Verification items for the finished model (mm, model axes). A direction names the side the tool comes from. Round coordinates to 2 decimals unless told otherwise and drop trailing zeros. Write each loop counter-clockwise with the first axis right and the second up, starting at its lowest first coordinate (ties: lowest second). Pieces come first, ordered by that corner, then holes. Notation, with made-up numbers: M 75,68 L 90,68 A25 ccw 90,85 Z; hole C -2,-28.5 d10. An arc over 180 degrees is marked long. One line per question, with ' | ' between items. Start each with the question number.
Q1. Cross-section at C-C (x = 86). Record the boundary of the cut face in (y, z).
Q2. Thickness scan on line 1 along X through (y, z) = (40, 11.3); line 2 along Y through (x, z) = (55, 12.5); line 3 along X through (y, z) = (88, 11.15). Record the ranges inside material, lowest first. Write a range as from..to.
Q3. Tool access check on faces 1 (the face through (172, 40, 5)), 2 (the face through (85, 76.5, 6)), 3 (the face through (101, 82, 10)). Record the directions out of +Z, -Z, +X, -X, +Y, -Y that give a thin tool (end or side, any length) a straight path to the whole face; none if there is none.
Q4. Cross-section at B-B (y = 40). Record the boundary of the cut face in (x, z).
Q5. Cross-section at A-A (x = 46). Record the boundary of the cut face in (y, z), then the cut area to 4 significant figures.
Q6. Gauge pin test, flat ends, axial feed: pin 1 (5 mm diameter, centred on y = 36.5, z = 5, fed in from -X); pin 2 (11 mm diameter, centred on x = 86, y = -8, fed in from -Z); pin 3 (1.5 mm diameter, centred on y = 55, z = 9, fed in from +X). Record the tip position at first contact, or that the pin passes through.
Q7. Cross-section at D-D (z = 5.75). Record the boundary of the cut face in (x, y), then the cut area to 4 significant figures.
Q8. Release check for a two-part mould opening along X. For faces 4 (the face through (85, 0, 5)), 5 (the face through (-13.15, 92.99, 11.52)), 6 (the face through (180, 40, 12)) record: released by +X, released by -X, zero draft, split by the parting line, or undercut.
from build123d import *

# Parameters (mm, degrees)
ESQUISSE1_W                  = 172
ESQUISSE1_H                  = 80
ESQUISSE1_W_2                = 165
ESQUISSE1_H_2                = 73
BOSS_EXTRU_1_DEPTH           = 10
ESQUISSE2_W                  = 204
ESQUISSE2_H                  = 112
ESQUISSE2_W_2                = 165
ESQUISSE2_H_2                = 73
BOSS_EXTRU_2_DEPTH           = 3
CONG_1_R                     = 10
CONG_2_R                     = 5
ENL_V_MAT_EXTRU_1_DEPTH      = 212.329127193
ENL_V_MAT_EXTRU_1_DEPTH_BACK = 2
ESQUISSE3_R                  = 3.5
ENL_V_MAT_EXTRU_2_DEPTH      = 212.492316645
ENL_V_MAT_EXTRU_2_DEPTH_BACK = 212.492316645
ESQUISSE4_R                  = 2
CHANFREIN1_SIZE              = 1.5


with BuildPart() as part:
    # Esquisse1 → Boss.-Extru.1 (new body)
    with BuildSketch(Plane.XY):
        with Locations((86, 40)):
            Rectangle(ESQUISSE1_W, ESQUISSE1_H)
        with Locations((86, 40)):
            Rectangle(ESQUISSE1_W_2, ESQUISSE1_H_2, mode=Mode.SUBTRACT)
    extrude(amount=BOSS_EXTRU_1_DEPTH)

    # Esquisse2 → Boss.-Extru.2 (add)
    with BuildSketch(Plane.XY.offset(10)):
        with Locations((86, 40)):
            Rectangle(ESQUISSE2_W, ESQUISSE2_H)
        with Locations((86, 40)):
            Rectangle(ESQUISSE2_W_2, ESQUISSE2_H_2, mode=Mode.SUBTRACT)
    extrude(amount=BOSS_EXTRU_2_DEPTH)

    # Congé1
    cong_1_edges = [part.edges().sort_by_distance(p)[0] for p in [
        (-16, 96, 11.5),
        (-16, -16, 11.5),
        (188, -16, 11.5),
        (188, 96, 11.5),
    ]]
    fillet(cong_1_edges, radius=CONG_1_R)

    # Congé2
    cong_2_edges = [part.edges().sort_by_distance(p)[0] for p in [
        (3.5, 76.5, 6.5),
        (3.5, 3.5, 6.5),
        (168.5, 3.5, 6.5),
        (168.5, 76.5, 6.5),
        (0, 80, 5),
        (172, 80, 5),
        (172, 0, 5),
        (0, 0, 5),
    ]]
    fillet(cong_2_edges, radius=CONG_2_R)

    # Esquisse3 → Enlèv. mat.-Extru.1 (cut, two sides: drawn at the far end of the back side and taken through both)
    with BuildSketch(Plane(origin=(0, 0, 10), x_dir=(-1, 0, 0), z_dir=(0, 0, -1)).offset(-ENL_V_MAT_EXTRU_1_DEPTH_BACK)):
        with Locations(Location((-180, 40, 0), (0, 0, 180))):
            Circle(ESQUISSE3_R)
        with Locations(Location((8, 40, 0), (0, 0, 180))):
            Circle(ESQUISSE3_R)
        with Locations(Location((-86, -8, 0), (0, 0, 180))):
            Circle(ESQUISSE3_R)
        with Locations(Location((-86, 88, 0), (0, 0, 180))):
            Circle(ESQUISSE3_R)
    extrude(amount=ENL_V_MAT_EXTRU_1_DEPTH + ENL_V_MAT_EXTRU_1_DEPTH_BACK, mode=Mode.SUBTRACT)

    # Esquisse4 → Enlèv. mat.-Extru.2 (cut, two sides: drawn at the far end of the back side and taken through both)
    with BuildSketch(Plane.XY.offset(13).offset(-ENL_V_MAT_EXTRU_2_DEPTH_BACK)):
        with Locations((-8, 70)):
            Circle(ESQUISSE4_R)
        with Locations((-8, 10)):
            Circle(ESQUISSE4_R)
        with Locations((180, 10)):
            Circle(ESQUISSE4_R)
        with Locations((180, 70)):
            Circle(ESQUISSE4_R)
        with Locations((46, 88)):
            Circle(ESQUISSE4_R)
        with Locations((126, 88)):
            Circle(ESQUISSE4_R)
        with Locations((126, -8)):
            Circle(ESQUISSE4_R)
        with Locations((46, -8)):
            Circle(ESQUISSE4_R)
    extrude(amount=ENL_V_MAT_EXTRU_2_DEPTH + ENL_V_MAT_EXTRU_2_DEPTH_BACK, mode=Mode.SUBTRACT)

    # Chanfrein1
    chanfrein1_edges = [part.edges().sort_by_distance(p)[0] for p in [
        (-10, 70, 13),
        (44, -8, 13),
        (124, -8, 13),
        (124, 88, 13),
        (44, 88, 13),
        (178, 70, 13),
        (178, 10, 13),
        (-10, 10, 13),
    ]]
    chamfer(chanfrein1_edges, length=CHANFREIN1_SIZE)


solid = part.part
Determined:
1) outline: M -16,10 L -11.5,10 L -11.5,12 L -4.5,12 L -4.5,10 L 0,10 L 0,0 L 3.5,0 L 3.5,13 L -16,13 Z; M 76.5,0 L 80,0 L 80,10 L 84.5,10 L 84.5,12 L 91.5,12 L 91.5,10 L 96,10 L 96,13 L 76.5,13 Z
2) line 1: x = -16..-11.5, -4.5..3.5, 168.5..176.5, 183.5..188 | line 2: y = -16..3.5, 76.5..96 | line 3: x = -15.8..44, 48..82.5, 89.5..124, 128..187.8
3) face 1: -Z, +X, +Y, -Y | face 2: +Z, -Z | face 3: -Z
4) outline: M -16,10 L -11.5,10 L -11.5,12 L -4.5,12 L -4.5,10 L 0,10 L 0,0 L 3.5,0 L 3.5,13 L -16,13 Z; M 168.5,0 L 172,0 L 172,10 L 176.5,10 L 176.5,12 L 183.5,12 L 183.5,10 L 188,10 L 188,13 L 168.5,13 Z
5) outline: M -16,10 L -10,10 L -10,11.5 L -11.5,13 L -16,13 Z; M -6,10 L 0,10 L 0,0 L 3.5,0 L 3.5,13 L -4.5,13 L -6,11.5 Z; M 76.5,0 L 80,0 L 80,10 L 86,10 L 86,11.5 L 84.5,13 L 76.5,13 Z; M 90,10 L 96,10 L 96,13 L 91.5,13 L 90,11.5 Z | area: 158.5 mm²
6) pin 1: stops at x = 0 | pin 2: stops at z = 10 | pin 3: stops at x = 172
7) outline: M 0,5 A5 ccw 5,0 L 167,0 A5 ccw 172,5 L 172,75 A5 ccw 167,80 L 5,80 A5 ccw 0,75 Z; hole M 3.5,8.5 A5 ccw 8.5,3.5 L 163.5,3.5 A5 ccw 168.5,8.5 L 168.5,71.5 A5 ccw 163.5,76.5 L 8.5,76.5 A5 ccw 3.5,71.5 Z | area: 1,715 mm²
8) face 4: zero draft | face 5: released by -X | face 6: undercut
